from build123d import *

# Parameters (mm, degrees)
ESTRUSIONE_ESTRUSIONE1_DEPTH = 2.5
ESTRUSIONE_ESTRUSIONE2_DEPTH = 15
SCHIZZO2_R                   = 10.25
SCHIZZO2_R_2                 = 2.8
TAGLIO_ESTRUSIONE1_DEPTH     = 15
SCHIZZO3_R                   = 16.1
SCHIZZO3_R_2                 = 14.5
ESTRUSIONE_ESTRUSIONE3_DEPTH = 0.5
SCHIZZO3_3_R                 = 18.6
SCHIZZO3_3_R_2               = 16.1
ESTRUSIONE_ESTRUSIONE4_DEPTH = 7.5
SCHIZZO3_4_R                 = 5
SCHIZZO3_4_R_2               = 2.8
ESTRUSIONE_ESTRUSIONE5_DEPTH = 6.1
SCHIZZO3_5_R                 = 6.3
SCHIZZO3_5_R_2               = 2.25
ESTRUSIONE_ESTRUSIONE6_DEPTH = 3.5
SMUSSO1_SIZE                 = 1.5
FORO_PER_VITE_M4_1_D         = 4.5
FORO_PER_VITE_M4_1_DEPTH     = 50
FORO_PER_VITE_M4_1_TIP       = 1.351936393


with BuildPart() as part:
    # Schizzo1 → Estrusione-Estrusione1 (new body)
    with BuildSketch(Plane.XY):
        with BuildLine():
            Line((5.123487201, 41.4), (126, 41.4))
            Line((126, 41.4), (126, -5.6))
            ThreePointArc((126, -5.6), (93.463092461, -9.435358059), (61.98889523, -18.531249019))
            Line((61.98889523, -18.531249019), (8.416056083, -38.9))
            ThreePointArc((8.416056083, -38.9), (-38.9, -8.416056083), (-8.416056083, 38.9))
            Line((-8.416056083, 38.9), (3.170362201, 41.207410603))
            ThreePointArc((3.170362201, 41.207410603), (4.142188579, 41.351736181), (5.123487201, 41.4))
        make_face()
    extrude(amount=ESTRUSIONE_ESTRUSIONE1_DEPTH)

    # Schizzo1<3> → Estrusione-Estrusione2 (add)
    with BuildSketch(Plane.XY):
        with BuildLine():
            Line((126, 41.4), (5.123487201, 41.4))
            ThreePointArc((5.123487201, 41.4), (4.142188579, 41.351736181), (3.170362201, 41.207410603))
            Line((3.170362201, 41.207410603), (-8.416056083, 38.9))
            ThreePointArc((-8.416056083, 38.9), (-38.9, -8.416056083), (8.416056083, -38.9))
            Line((8.416056083, -38.9), (61.98889523, -18.531249019))
            ThreePointArc((61.98889523, -18.531249019), (93.463092461, -9.435358059), (126, -5.6))
            Line((126, -5.6), (126, -3.098457484))
            ThreePointArc((126, -3.098457484), (91.357291517, -7.317073844), (57.953366675, -17.421121553))
            Line((57.953366675, -17.421121553), (7.887409345, -36.456532663))
            ThreePointArc((7.887409345, -36.456532663), (-36.58362067, -7.275211244), (-6.660968885, 36.700429065))
            Line((-6.660968885, 36.700429065), (3.41687663, 38.707410603))
            ThreePointArc((3.41687663, 38.707410603), (4.388703008, 38.851736181), (5.37000163, 38.9))
            Line((5.37000163, 38.9), (126, 38.9))
            Line((126, 38.9), (126, 41.4))
        make_face()
    extrude(amount=ESTRUSIONE_ESTRUSIONE2_DEPTH)

    # Schizzo2 → Taglio-Estrusione1 (cut)
    with BuildSketch(Plane(origin=(0, 0, 0), x_dir=(-1, 0, 0), z_dir=(0, 0, -1))):
        Circle(SCHIZZO2_R)
        with Locations((0, -26)):
            Circle(SCHIZZO2_R_2)
        with Locations((26, 0)):
            Circle(SCHIZZO2_R_2)
        with Locations((0, 26)):
            Circle(SCHIZZO2_R_2)
    extrude(amount=-TAGLIO_ESTRUSIONE1_DEPTH, mode=Mode.SUBTRACT)

    # Schizzo3 → Estrusione-Estrusione3 (add)
    with BuildSketch(Plane.XY.offset(2.5)):
        Circle(SCHIZZO3_R)
        Circle(SCHIZZO3_R_2, mode=Mode.SUBTRACT)
    extrude(amount=ESTRUSIONE_ESTRUSIONE3_DEPTH)

    # Schizzo3<3> → Estrusione-Estrusione4 (add)
    with BuildSketch(Plane.XY.offset(2.5)):
        Circle(SCHIZZO3_3_R)
        Circle(SCHIZZO3_3_R_2, mode=Mode.SUBTRACT)
    extrude(amount=ESTRUSIONE_ESTRUSIONE4_DEPTH)

    # Schizzo3<4> → Estrusione-Estrusione5 (add)
    # profile 1 of 4: a face of its own
    with BuildSketch(Plane.XY.offset(2.5)):
        with Locations((-26, 0)):
            Circle(SCHIZZO3_4_R)
        with Locations(Location((-26, 0, 0), (0, 0, 180))):
            Circle(SCHIZZO3_4_R_2, mode=Mode.SUBTRACT)
    # profile 2 of 4: a face of its own
    with BuildSketch(Plane.XY.offset(2.5)):
        with Locations((0, -26)):
            Circle(SCHIZZO3_4_R)
        with Locations(Location((0, -26, 0), (0, 0, 180))):
            Circle(SCHIZZO3_4_R_2, mode=Mode.SUBTRACT)
    # profile 3 of 4: a face of its own
    with BuildSketch(Plane.XY.offset(2.5)):
        with Locations((26, 0)):
            Circle(SCHIZZO3_4_R)
        with Locations((26, 0)):
            Circle(SCHIZZO3_4_R_2, mode=Mode.SUBTRACT)
    # profile 4 of 4: a face of its own
    with BuildSketch(Plane.XY.offset(2.5)):
        with Locations((0, 26)):
            Circle(SCHIZZO3_4_R)
        with Locations(Location((0, 26, 0), (0, 0, 180))):
            Circle(SCHIZZO3_4_R_2, mode=Mode.SUBTRACT)
    extrude(amount=ESTRUSIONE_ESTRUSIONE5_DEPTH)

    # Schizzo3<5> → Estrusione-Estrusione6 (add)
    # profile 1 of 2: a face of its own
    with BuildSketch(Plane.XY.offset(2.5)):
        with Locations((55, 17.9)):
            Circle(SCHIZZO3_5_R)
        with Locations((55, 17.9)):
            Circle(SCHIZZO3_5_R_2, mode=Mode.SUBTRACT)
    # profile 2 of 2: a face of its own
    with BuildSketch(Plane.XY.offset(2.5)):
        with Locations((101, 17.9)):
            Circle(SCHIZZO3_5_R)
        with Locations((101, 17.9)):
            Circle(SCHIZZO3_5_R_2, mode=Mode.SUBTRACT)
    extrude(amount=ESTRUSIONE_ESTRUSIONE6_DEPTH)

    # Smusso1
    # the kernel refuses this chamfer: 1.5 mm, written as the material it adds along each edge
    with BuildSketch(Plane(origin=(0, 0, 2.5), x_dir=(1, 0, 0), z_dir=(0, -1, 0))) as smusso1_piece_1:
        Polygon((18.6 + SMUSSO1_SIZE, 0), (18.6, SMUSSO1_SIZE), (18.6, 0), align=None)
    revolve(axis=Axis((0, 0, 2.5), (0, 0, 1)))
    with BuildSketch(Plane(origin=(-26, 0, 2.5), x_dir=(1, 0, 0), z_dir=(0, -1, 0))) as smusso1_piece_2:
        Polygon((5 + SMUSSO1_SIZE, 0), (5, SMUSSO1_SIZE), (5, 0), align=None)
    revolve(axis=Axis((-26, 0, 2.5), (0, 0, 1)))
    with BuildSketch(Plane(origin=(0, -26, 2.5), x_dir=(1, 0, 0), z_dir=(0, -1, 0))) as smusso1_piece_3:
        Polygon((5 + SMUSSO1_SIZE, 0), (5, SMUSSO1_SIZE), (5, 0), align=None)
    revolve(axis=Axis((0, -26, 2.5), (0, 0, 1)))
    with BuildSketch(Plane(origin=(26, 0, 2.5), x_dir=(1, 0, 0), z_dir=(0, -1, 0))) as smusso1_piece_4:
        Polygon((5 + SMUSSO1_SIZE, 0), (5, SMUSSO1_SIZE), (5, 0), align=None)
    revolve(axis=Axis((26, 0, 2.5), (0, 0, 1)))
    with BuildSketch(Plane(origin=(0, 26, 2.5), x_dir=(1, 0, 0), z_dir=(0, -1, 0))) as smusso1_piece_5:
        Polygon((5 + SMUSSO1_SIZE, 0), (5, SMUSSO1_SIZE), (5, 0), align=None)
    revolve(axis=Axis((0, 26, 2.5), (0, 0, 1)))
    # the kernel refuses this chamfer: 1.5 mm, written as the material it takes off along each edge
    with BuildSketch(Plane(origin=(55, 17.9, 6), x_dir=(1, 0, 0), z_dir=(0, -1, 0))) as smusso1_2_piece_1:
        Polygon((6.3, -SMUSSO1_SIZE), (6.3 - SMUSSO1_SIZE, 0), (6.3, 0), align=None)
    revolve(axis=Axis((55, 17.9, 6), (0, 0, 1)), mode=Mode.SUBTRACT)
    with BuildSketch(Plane(origin=(101, 17.9, 6), x_dir=(1, 0, 0), z_dir=(0, -1, 0))) as smusso1_2_piece_2:
        Polygon((6.3, -SMUSSO1_SIZE), (6.3 - SMUSSO1_SIZE, 0), (6.3, 0), align=None)
    revolve(axis=Axis((101, 17.9, 6), (0, 0, 1)), mode=Mode.SUBTRACT)

    # Foro per Vite M4-1
    with Locations(Plane(origin=(55, 17.9, 0), x_dir=(-1, 0, 0), z_dir=(0, 0, -1))):
        with Locations((0, 0), (-46, 0)):
            Hole(FORO_PER_VITE_M4_1_D / 2, depth=FORO_PER_VITE_M4_1_DEPTH)
            with Locations((0, 0, -(FORO_PER_VITE_M4_1_DEPTH + FORO_PER_VITE_M4_1_TIP / 2))):  # 118° drill point
                Cone(0, FORO_PER_VITE_M4_1_D / 2, FORO_PER_VITE_M4_1_TIP, mode=Mode.SUBTRACT)


solid = part.part
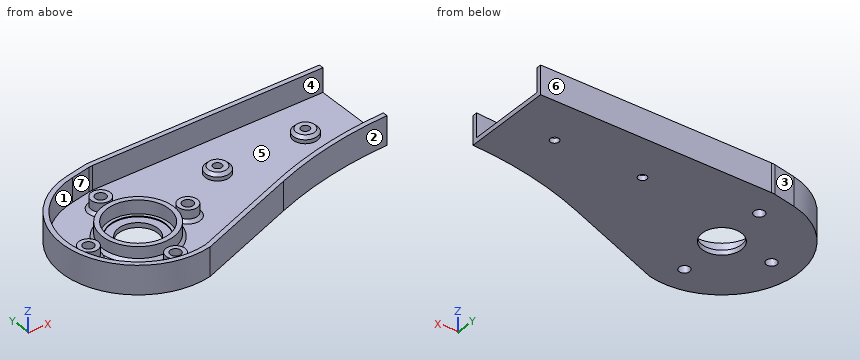
For this review, take the finished solid that the model builds, in its own axes (mm). Face numbers are marked on the shaded views. A direction names the side the tool comes from. Coordinates: 2 decimals unless noted, no trailing zeros. Loops run counter-clockwise (first coordinate to the right, second up) from the corner with the lowest first, then second, coordinate; pieces in that order, holes last. Notation, with made-up numbers: (57.5, 84) - (74.5, 84) arc R17 cw to (74.5, 106) - close; hole circle Ø8 at (10, 9). An arc over 180 degrees is marked (long way). Use a Markdown table: item, result. Add a question column.
Item 1: We need section A-A (y = 26). Give the boundary of the cut face in (x, z), and give its area (3 significant figures).
Item 2: Insertion check: pin 1 Ø3 at (x, z) = (22.5, 13) entering from -Y; pin 2 Ø1.5 at (x, y) = (-19, -22.5) entering from +Z; pin 3 Ø4.5 at (x, y) = (0, 26) entering from -Z; pin 4 Ø7.5 at (x, y) = (57, 19.5) entering from +Z. Each pin has a flat end and moves straight along its axis. Give the tip position at first contact, or say it passes through.
Item 3: We need section C-C (z = 11.75). Give the boundary of the cut face in (x, y), and give its area (3 significant figures).
Item 4: For line 1 (X direction, y = 24.5, z = 6); line 2 (Y direction, x = -26, z = 5.25); line 3 (X direction, y = 14.5, z = 4.75), list the stretches that pass through material, from the lowest coordinate up.
Item 5: Tool access review of the marked faces 5, 6 and 7: name each direction out of +Z, -Z, +X, -X, +Y, -Y from which nothing blocks a thin tool from reaching the whole face with its end or side.
Item 6: We need section D-D (y = 0). Give the number of separate pieces and of enclosed holes in the cut face, and give its area (3 significant figures).
Item 7: Mouldability with a two-part tool opening along X and no side actions: class the marked faces 1, 2, 3 and 4 as pulls with the +X half, pulls with the -X half, needs draft (parallel to the pull), parting line crosses it, or undercut.
Item 8: We need section B-B (x = 55). Give the boundary of the cut face in (y, z).
Results list:
| question | item | result |
|---|---|---|
| 1 | outline | (-30.13, 0) - (-2.8, 0) - (-2.8, 8.6) - (-5, 8.6) - (-5, 4) - (-6.5, 2.5) - (-26.74, 2.5) - (-26.74, 15) - (-30.13, 15) - close; (2.8, 0) - (126, 0) - (126, 2.5) - (6.5, 2.5) - (5, 4) - (5, 8.6) - (2.8, 8.6) - close |
| 1 | area | 448 mm^2 |
| 2 | pin 1 | stops at y = -34.12 |
| 2 | pin 2 | stops at z = 2.5 |
| 2 | pin 3 | passes through |
| 2 | pin 4 | stops at z = 6 |
| 3 | outline | (-8.42, 38.9) arc R39.8 ccw to (8.42, -38.9) - (61.99, -18.53) arc R200 cw to (126, -5.6) - (126, -3.1) arc R202.5 ccw to (57.95, -17.42) - (7.89, -36.46) arc R37.3 cw (long way) to (-6.66, 36.7) - (3.42, 38.71) arc R10 cw to (5.37, 38.9) - (126, 38.9) - (126, 41.4) - (5.12, 41.4) arc R10 ccw to (3.17, 41.21) - close |
| 3 | area | 945 mm^2 |
| 4 | line 1 | x = -31.37 to -28.13, -4.77 to -2.36, 2.36 to 4.77 |
| 4 | line 2 | y = -30.13 to -26.74, -5 to -2.8, 2.8 to 5, 26.74 to 30.13 |
| 4 | line 3 | x = -37.06 to -34.37, -11.65 to -7, 7 to 11.65, 50 to 60, 96 to 106 |
| 5 | face 5 | +Z |
| 5 | face 6 | +Z, -Z, +X, -X, +Y |
| 5 | face 7 | +Z, +X |
| 6 | separate pieces | 3 |
| 6 | enclosed holes | 0 |
| 6 | area | 480 mm^2 |
| 7 | face 1 | undercut |
| 7 | face 2 | pulls with the +X half |
| 7 | face 3 | pulls with the -X half |
| 7 | face 4 | needs draft |
| 8 | outline | (-21.19, 0) - (15.65, 0) - (15.65, 6) - (13.1, 6) - (11.6, 4.5) - (11.6, 2.5) - (-18.54, 2.5) - (-18.54, 15) - (-21.19, 15) - close; (20.15, 0) - (41.4, 0) - (41.4, 15) - (38.9, 15) - (38.9, 2.5) - (24.2, 2.5) - (24.2, 4.5) - (22.7, 6) - (20.15, 6) - close |
